Could you check a few things on this model? Use its own coordinates, in mm. A direction names the side the tool comes from. Round coordinates to 2 decimals unless told otherwise and drop trailing zeros. Loops run counter-clockwise (first coordinate to the right, second up) from the corner with the lowest first, then second, coordinate; pieces in that order, holes last. Notation, with made-up numbers: (6, -20.75) -> (55, -20.75) arc R22 ccw to (55, 11.25) -> close; hole circle Ø10 at (47.5, 84.25). An arc over 180 degrees is marked (long way). Use CSV: the item, a comma, the result in double quotes. Start each with the question number.
```python
from build123d import *

# Parameters (mm, degrees)
BOSS_EXTRUDE1_DEPTH                            = 6
BOSS_EXTRUDE2_DEPTH                            = 14.89
BOSS_EXTRUDE3_DEPTH                            = 14.89
CBORE_FOR_6_SOCKET_HEAD_CAP_SCREW1_D           = 3.7973
CBORE_FOR_6_SOCKET_HEAD_CAP_SCREW1_CBORE_D     = 7.14502
CBORE_FOR_6_SOCKET_HEAD_CAP_SCREW1_CBORE_DEPTH = 3.5052
F_6_CLEARANCE_HOLE1_D                          = 3.7973
FILLET1_R                                      = 5
FILLET2_R                                      = 5
FILLET3_R                                      = 2
F_6_CLEARANCE_HOLE2_D                          = 3.7973


with BuildPart() as part:
    # Sketch1 → Boss-Extrude1 (new body)
    with BuildSketch(Plane.XY):
        with BuildLine():
            ThreePointArc((76.2635, 0), (-29.032526712, 70.521158704), (-54.158886199, -53.692983507))
            Line((-54.158886199, -53.692983507), (-40.58534353, -40.236207458))
            ThreePointArc((-40.58534353, -40.236207458), (-21.756264814, 52.846830003), (57.15, 0))
            ThreePointArc((57.15, 0), (52.846830003, -21.756264814), (40.58534353, -40.236207458))
            Line((40.58534353, -40.236207458), (54.158886199, -53.692983507))
            ThreePointArc((54.158886199, -53.692983507), (70.521158704, -29.032526712), (76.2635, 0))
        make_face()
        with BuildLine():
            ThreePointArc((30, 83.685183874), (0, 88.9), (-30, 83.685183874))
            ThreePointArc((-30, 83.685183874), (-85.211894281, 25.340542083), (-70.853888546, -53.692983507))
            Line((-70.853888546, -53.692983507), (-54.158886199, -53.692983507))
            ThreePointArc((-54.158886199, -53.692983507), (-29.032526712, 70.521158704), (76.2635, 0))
            ThreePointArc((76.2635, 0), (70.521158704, -29.032526712), (54.158886199, -53.692983507))
            Line((54.158886199, -53.692983507), (70.853888546, -53.692983507))
            ThreePointArc((70.853888546, -53.692983507), (84.267789492, -28.322246629), (88.9, 0))
            ThreePointArc((88.9, 0), (72.698727637, 51.167421276), (30, 83.685183874))
        make_face()
    extrude(amount=BOSS_EXTRUDE1_DEPTH)

    # Sketch1_3 → Boss-Extrude2 (add)
    with BuildSketch(Plane.XY):
        with BuildLine():
            ThreePointArc((30, 83.685183874), (0, 88.9), (-30, 83.685183874))
            ThreePointArc((-30, 83.685183874), (-85.211894281, 25.340542083), (-70.853888546, -53.692983507))
            Line((-70.853888546, -53.692983507), (-54.158886199, -53.692983507))
            ThreePointArc((-54.158886199, -53.692983507), (-29.032526712, 70.521158704), (76.2635, 0))
            ThreePointArc((76.2635, 0), (70.521158704, -29.032526712), (54.158886199, -53.692983507))
            Line((54.158886199, -53.692983507), (70.853888546, -53.692983507))
            ThreePointArc((70.853888546, -53.692983507), (84.267789492, -28.322246629), (88.9, 0))
            ThreePointArc((88.9, 0), (72.698727637, 51.167421276), (30, 83.685183874))
        make_face()
    extrude(amount=BOSS_EXTRUDE2_DEPTH)

    # Sketch1_4 → Boss-Extrude3 (add)
    with BuildSketch(Plane.XY):
        with BuildLine():
            Line((-30, 93.594750756), (-30, 83.685183874))
            ThreePointArc((-30, 83.685183874), (0, 88.9), (30, 83.685183874))
            Line((30, 83.685183874), (30, 93.594750756))
            ThreePointArc((30, 93.594750756), (0, 98.285183874), (-30, 93.594750756))
        make_face()
    extrude(amount=BOSS_EXTRUDE3_DEPTH)

    # CBORE for _6 Socket Head Cap Screw1 (through all)
    with Locations(Plane(origin=(74.81570782, -34.887137507, 0), x_dir=(-1, 0, 0), z_dir=(0, 0, -1))):
        with Locations((0, 0), (11.578739041, 87.949254687), (138.052676599, 87.949254687), (149.63141564, 0)):
            CounterBoreHole(CBORE_FOR_6_SOCKET_HEAD_CAP_SCREW1_D / 2, CBORE_FOR_6_SOCKET_HEAD_CAP_SCREW1_CBORE_D / 2, CBORE_FOR_6_SOCKET_HEAD_CAP_SCREW1_CBORE_DEPTH)

    # 6 Clearance Hole1 (through all)
    with Locations(Plane(origin=(0, 88, 14.89), x_dir=(1, 0, 0), z_dir=(0, 0, 1))):
        with Locations((0, 0), (20.32, 0), (-20.32, 0)):
            Hole(F_6_CLEARANCE_HOLE1_D / 2)

    # Fillet1
    fillet1_edges = [part.edges().sort_by_distance(p)[0] for p in [
        (30, 83.685183874, 7.445),
        (-30, 83.685183874, 7.445),
    ]]
    fillet(fillet1_edges, radius=FILLET1_R)

    # Fillet2
    fillet2_edges = [part.edges().sort_by_distance(p)[0] for p in [
        (30, 93.594750756, 7.445),
        (-30, 93.594750756, 7.445),
    ]]
    fillet(fillet2_edges, radius=FILLET2_R)

    # Fillet3
    fillet3_edges = [part.edges().sort_by_distance(p)[0] for p in [
        (30.857632087, 84.333147978, 0),
        (0, 98.285183874, 0),
        (28.981198623, 92.897735968, 0),
        (-28.981198623, 92.897735968, 0),
        (-70.853888546, -53.692983507, 7.445),
        (70.853888546, -53.692983507, 7.445),
        (-47.372114864, -46.964595482, 0),
        (-62.506387373, -53.692983507, 0),
        (85.674892695, 23.728100677, 0),
        (62.506387373, -53.692983507, 0),
        (47.372114864, -46.964595482, 0),
        (-21.756264814, 52.846830003, 0),
        (-85.674892695, 23.728100677, 0),
        (-30, 88.503059235, 0),
        (30, 88.503059235, 0),
        (-30.857632087, 84.333147978, 0),
    ]]
    fillet(fillet3_edges, radius=FILLET3_R)

    # 6 Clearance Hole2 (through all)
    with Locations(Plane(origin=(62.559596708, -36.1188, 0), x_dir=(-1, 0, 0), z_dir=(0, 0, -1))):
        with Locations((0, 0), (0, 72.2376), (62.559596708, 108.3564), (125.119193416, 72.2376), (125.119193416, 0)):
            Hole(F_6_CLEARANCE_HOLE2_D / 2)


solid = part.part
```
1. For faces 1 (the face through (61.316, 56.074, 1.728)), 2 (the face through (61.73, 51.91, 9.28)), 3 (the face through (-17, 55, 6)), 4 (the face through (-47.7, -46.44, 0.57)), which set-ups out of +Z, -Z, +X, -X, +Y, -Y let a thin tool reach every point of the face, with its end or its side?
2. Will these pins go through, and if not, where does the flat tip stop? pin 1 (1.4 mm diameter, centred on y = 88, z = 10, fed in from +X); pin 2 (2 mm diameter, centred on x = 75.5, y = -33.5, fed in from -Z); pin 3 (2.5 mm diameter, centred on x = 63.24, y = 53.06, fed in from -Z); pin 4 (4 mm diameter, centred on x = 38.5, z = 6, fed in from -Y).
3. If I drill on L1, parallel to X at y = 0, z = 4.7; L2, parallel to X at y = 88, z = 5.75; L3, parallel to Y at x = 0, z = 8.5, over which ranges is the centre line in solid material (lowest first)?
4. Suppose I cut it at B-B (x = 0). State how many separate pieces and enclosed holes the cut face has, then the cut area to 3 significant figures.
5. We'd pull the mould along X, two halves only. Please class faces 5 (the face through (-78.116, -36.255, 1.728)), 6 (the face through (0, 79, 14.89)), 7 (the face through (0.373, 98.284, 8.355)), 8 (the face through (76.57, -35.61, 9.28)): pulls with the +X half, pulls with the -X half, needs draft (parallel to the pull), parting line crosses it, or undercut.
6. Suppose I cut it at A-A (z = 10.75). List the corners of the cut face in (x, y) for me.
Geometry check:
1,face 1,"-Z"
1,face 2,"+Z, -Z"
1,face 3,"+Z"
1,face 4,"-Z, -Y"
2,pin 1,"stops at x = 30"
2,pin 2,"stops at z = 3.51"
2,pin 3,"passes through"
2,pin 4,"stops at y = 40.32"
3,L1,"x = -88.9 to -57.15, 57.15 to 88.9"
3,L2,"x = -30 to -22.22, -18.42 to -1.9, 1.9 to 18.42, 22.22 to 30"
3,L3,"y = 76.26 to 86.1, 89.9 to 98.29"
4,separate pieces,"3"
4,enclosed holes,"0"
4,area,"362 mm²"
5,face 5,"undercut"
5,face 6,"needs draft"
5,face 7,"parting line crosses it"
5,face 8,"undercut"
6,outline,"(-71.46, -52.88) arc R2 ccw to (-69.85, -53.69) -> (-54.16, -53.69) arc R76.26 cw (long way) to (54.16, -53.69) -> (69.85, -53.69) arc R2 ccw to (71.46, -52.88) arc R88.9 ccw to (33.14, 82.49) arc R5 cw to (30, 87.13) -> (30, 89.87) arc R5 ccw to (26.34, 94.69) arc R98.29 ccw to (-26.34, 94.69) arc R5 ccw to (-30, 89.87) -> (-30, 87.13) arc R5 cw to (-33.14, 82.49) arc R88.9 ccw to start; hole circle Ø3.8 at (-74.82, -34.89); hole circle Ø3.8 at (-63.24, 53.06); hole circle Ø3.8 at (-20.32, 88); hole circle Ø3.8 at (0, 88); hole circle Ø3.8 at (20.32, 88); hole circle Ø3.8 at (63.24, 53.06); hole circle Ø3.8 at (74.82, -34.89)"
